For this review, take the finished solid that the model builds, in its own axes (mm). A direction names the side the tool comes from. Give positions to 0.01 mm unless a question says otherwise; leave off trailing zeros. Write each loop counter-clockwise with the first axis right and the second up, starting at its lowest first coordinate (ties: lowest second). Pieces come first, ordered by that corner, then holes.
Q1. We need section A-A (z = -27.5). Write out the cut boundary in (x, y).
Q2. For line 1 (Z direction, x = 20, y = 5); line 2 (X direction, y = 8.25, z = -10); line 3 (X direction, y = 2.25, z = -54.5), list the stretches that pass through material, from the lowest coordinate up.
Q3. Machinability: for faces 4 (the flat face through (118.65, 2, -47)), 5 (the flat face through (122.65, 2, -35)), 6 (the cylindrical face through (19.62, 6.45, -59.11)), which of the approach directions +Z, -Z, +X, -X, +Y, -Y give a long, thin tool a straight path to every point of the face, cutting with its end or side? Answer none if there is none.
Q4. We need section B-B (x = 48). Write out the cut boundary in (y, z).
Q5. Mouldability with a two-part tool opening along X and no side actions: class faces 1 (the flat face through (18, 2, -35)), 2 (the flat face through (19, 10, -59)), 3 (the cylindrical face through (21.846, 4.93, -63.849)) as released by +X, released by -X, zero draft, split by the parting line, or undercut.
Q6. Insertion check: P1, Ø2, axis at y = 1.5, z = -27, coming from the +X side; P2, Ø6, axis at x = 64, y = 6.5, coming from the -Z side; P3, Ø2, axis at x = 61, y = 2.5, coming from the +Z side; P4, Ø12, axis at x = 97, z = -26.5, coming from the +Y side. Each pin has a flat end and moves straight along its axis. Give the tip position at first contact, or say it passes through.
Autodesk Fusion 360 part; units mm, degrees
sketch "Schizzo7" plane through (0, 0, 0) normal (0, 1, 0) x (1, 0, 0)
  line L0 (20, 10) -> (120.65, 10)
  line L1 (120.65, 10) -> (120.65, 60.3)
  line L2 (120.65, 60.3) -> (20, 60.3)
  line L3 (20, 60.3) -> (20, 10)
  circle A0 centre (120.65, 60.3) radius 4
  circle A1 centre (20, 60.3) radius 4
  circle A2 centre (20, 10) radius 4
  circle A3 centre (120.65, 10) radius 4
  line L4 (20, 60.3) -> (18, 60.3)
  line L5 (18, 60.3) -> (20, 60.3)
  line L6 (20, 60.3) -> (22, 60.3)
  line L7 (22, 60.3) -> (22, 10)
  line L8 (18, 60.3) -> (18, 10)
  line L9 (120.65, 60.3) -> (122.65, 60.3)
  line L10 (120.65, 60.3) -> (118.65, 60.3)
  line L11 (118.65, 60.3) -> (118.65, 10)
  line L12 (122.65, 60.3) -> (122.65, 10)
  line L13 (122.65, 10) -> (120.65, 10)
  line L14 (20, 35.15) -> (120.65, 35.15)
  line L15 (22, 35.15) -> (22, 37.65)
  line L16 (22, 35.15) -> (22, 32.65)
  line L17 (22, 37.65) -> (118.65, 37.65)
  line L18 (22, 32.65) -> (118.65, 32.65)
  dimension "d45" = 100.65
  dimension "d46" = 50.3
  dimension "d47" = 8
  dimension "d48" = 8
  dimension "d49" = 8
  dimension "d50" = 8
  dimension "d51" = 2
  dimension "d52" = 2
  dimension "d53" = 2.5
  dimension "d54" = 2.5
extrude "Estrusione12" add sketch "Schizzo7" along normal blind 4 contours L3 A1 A2 L8 | L3 A2 L7 L14 L16 | L3 A1 L7 L14 L15 | L7 L11 L14 L16 L18 | L7 L11 L14 L15 L17 | L1 A3 L11 L14 | L1 A0 L11 L14 | L1 A0 A3 L12
extrude "Estrusione13" add sketch "Schizzo7" along normal blind 10 contours L0 L3 A2 L7 | L0 L3 A2 | L0 A2 L7 | L0 A3 L11 | L0 A3 L12 L13 | L3 A1 L4 L5 L8 | L2 L3 A1 L6 L7 | L2 A1 L4 L5 L6 L8 | L0 L1 A3 L11 | L2 A1 L7 | L1 A3 L12 L13 | L2 A0 L9 L10 L12 | L2 A0 L11 | L1 A0 L9 L12 | L1 L2 A0 L10 L11
hole "Foratura1" at (120.65, 10, -60.3) direction (0, -1, 0) diameter 2.5 depth 7 tip angle 118
hole "Foratura2" at (120.65, 10, -10) direction (0, -1, 0) diameter 2.5 depth 7 tip angle 118
hole "Foratura3" at (20, 10, -10) direction (0, -1, 0) diameter 2.5 depth 7 tip angle 118
hole "Foratura4" at (20, 10, -60.3) direction (0, -1, 0) diameter 2.5 depth 7 tip angle 118
Computed:
1. outline: (18, 0) - (22, 0) - (22, 4) - (18, 4) - close; (118.65, 0) - (122.65, 0) - (122.65, 4) - (118.65, 4) - close
2. line 1: z = -64.3 to -61.55, -59.05 to -56.3, -14 to -11.25, -8.75 to -6
2. line 2: x = 16 to 18.75, 21.25 to 24, 116.65 to 119.4, 121.9 to 124.65
2. line 3: x = 18 to 22, 118.65 to 122.65
3. face 4: +Y, -Y
3. face 5: +X, +Y, -Y
3. face 6: +Y
4. outline: (0, -37.65) - (4, -37.65) - (4, -32.65) - (0, -32.65) - close
5. face 1: released by -X
5. face 2: zero draft
5. face 3: undercut
6. P1: stops at x = 122.65
6. P2: stops at z = -37.65
6. P3: stops at z = -32.65
6. P4: passes through
